The listing builds one solid part. Answer for the finished solid, in the listing's coordinates (mm). Face numbers are marked on the shaded views. A direction names the side the tool comes from. Round coordinates to 2 decimals unless told otherwise and drop trailing zeros. Write each loop counter-clockwise with the first axis right and the second up, starting at its lowest first coordinate (ties: lowest second). Pieces come first, ordered by that corner, then holes.
from build123d import *
from build123d.topology import SkipClean

# Parameters (mm, degrees)
EXTRUDE_1_DEPTH = 4
SKETCH_2_R      = 3
SKETCH_2_R_2    = 1.05
EXTRUDE_2_DEPTH = 3
EXTRUDE_START   = -7
SKETCH_3_R      = 2
EXTRUDE_3_DEPTH = 7


with BuildPart() as part:
    # Эскиз1 → Бобышка-Вытянуть1 (new body)
    with BuildSketch(Plane.XY):
        with BuildLine():
            Line((14.386891947, -11.67121845), (-1.44161316, -9.187586816))
            ThreePointArc((-1.44161316, -9.187586816), (-8.668259234, 3.369166345), (5.141479906, 7.74952801))
            Line((5.141479906, 7.74952801), (18.492476869, -1.108286623))
            ThreePointArc((18.492476869, -1.108286623), (20.691973654, -8.042526113), (14.386891947, -11.67121845))
        make_face()
        with BuildLine():
            Line((3.482938001, 5.249680265), (16.833934964, -3.608134368))
            ThreePointArc((16.833934964, -3.608134368), (17.895760998, -6.95569826), (14.85192845, -8.707480768))
            Line((14.85192845, -8.707480768), (-0.976576656, -6.223849133))
            ThreePointArc((-0.976576656, -6.223849133), (-5.872046578, 2.282338492), (3.482938001, 5.249680265))
        make_face(mode=Mode.SUBTRACT)
    extrude(amount=EXTRUDE_1_DEPTH)

    # Эскиз2 → Бобышка-Вытянуть2 (add)
    with SkipClean():  # the faces are left unmerged after this step: merging them gives an invalid solid
        with BuildSketch(Plane.XY.offset(4)):
            with BuildLine():
                Line((-1.44161316, -9.187586816), (14.386891947, -11.67121845))
                ThreePointArc((14.386891947, -11.67121845), (20.691973654, -8.042526113), (18.492476869, -1.108286623))
                Line((18.492476869, -1.108286623), (5.141479906, 7.74952801))
                ThreePointArc((5.141479906, 7.74952801), (-8.668259234, 3.369166345), (-1.44161316, -9.187586816))
            make_face()
            Circle(SKETCH_2_R, mode=Mode.SUBTRACT)
            with Locations((6.897324552, -2.680842038)):
                Circle(SKETCH_2_R_2, mode=Mode.SUBTRACT)
            with Locations((9.693537208, -3.767669891)):
                Circle(SKETCH_2_R_2, mode=Mode.SUBTRACT)
            with Locations((12.489749864, -4.854497744)):
                Circle(SKETCH_2_R_2, mode=Mode.SUBTRACT)
            with Locations((15.28596252, -5.941325597)):
                Circle(SKETCH_2_R_2, mode=Mode.SUBTRACT)
        extrude(amount=EXTRUDE_2_DEPTH)

    # Эскиз3 → Бобышка-Вытянуть3 (add)
    with SkipClean():  # the faces are left unmerged after this step: merging them gives an invalid solid
        with BuildSketch(Plane.XY.offset(7).offset(EXTRUDE_START)):
            with BuildLine():
                Line((18.492476869, -1.108286623), (24.987431668, -4.371825212))
                ThreePointArc((24.987431668, -4.371825212), (27.402884029, -10.650912961), (21.380978505, -13.650580764))
                Line((21.380978505, -13.650580764), (14.386891947, -11.67121845))
                ThreePointArc((14.386891947, -11.67121845), (20.691973654, -8.042526113), (18.492476869, -1.108286623))
            make_face()
            with Locations((22.742529602, -8.839533206)):
                Circle(SKETCH_3_R, mode=Mode.SUBTRACT)
        extrude(amount=EXTRUDE_3_DEPTH)


solid = part.part
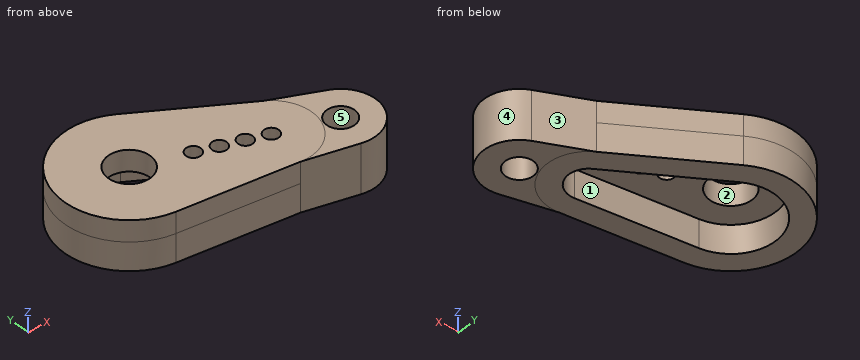
1. Section C-C on z = 2.25 is taken. Determine the outline of the cut face in (x, y).
Geometry says:
outline: (-1.44, -9.19) - (14.39, -11.67) - (21.38, -13.65) arc R5 ccw to (24.99, -4.37) - (18.49, -1.11) - (5.14, 7.75) arc R9.3 ccw (long way) to start; hole (-0.98, -6.22) - (14.85, -8.71) arc R2.8 ccw to (16.83, -3.61) - (3.48, 5.25) arc R6.3 ccw (long way) to start; hole circle Ø4 at (22.74, -8.84)
2. A tool of negligible diameter and unlimited length cuts with its end or side. For the marked faces 1 and 2, from which of +Z, -Z, +X, -X, +Y, -Y can it reach the whole face along a straight path? Write none if from no direction.
Geometry says:
face 1: -Z
face 2: +Z, -Z
3. Section B-B on y = -8 is taken. Determine the outline of the cut face in (x, z).
Geometry says:
outline: (-4.74, 0) - (10.34, 0) - (10.34, 4) - (17.18, 4) - (17.18, 0) - (20.93, 0) - (20.93, 7) - (-4.74, 7) - close; (24.56, 0) - (27.67, 0) - (27.67, 7) - (24.56, 7) - close
4. Given pin 1 (2.5 mm diameter, centred on x = 12.49, y = -4.85, fed in from -Z); pin 2 (1.7 mm diameter, centred on x = 9.69, y = -3.77, fed in from -Z); pin 3 (1.5 mm diameter, centred on x = 13, z = 2, fed in from +Y); pin 4 (1 mm diameter, centred on x = 11, z = 5.5, fed in from -Y), each flat-ended and moving along its own axis, determine where each tip first touches the part or whether it passes through.
Geometry says:
pin 1: stops at z = 4
pin 2: passes through
pin 3: stops at y = 3.03
pin 4: stops at y = -11.22
5. Straight lines are drawn through the part: line 1 along X through (y, z) = (-4.75, 1.25); line 2 along X through (y, z) = (-5.5, 2); line 3 along Z through (x, y) = (7.5, -5.75). For each, find the intervals that lie inside material, in ascending order.
Geometry says:
line 1: x = -8 to -4.14, 17.82 to 25.62
line 2: x = -7.5 to -3.07, 18.05 to 26.46
line 3: z = 4 to 7
6. Section A-A on x = 0 is taken. Determine the outline of the cut face in (y, z), plus the area to 3 significant figures.
Geometry says:
outline: (-9.41, 0) - (-6.38, 0) - (-6.38, 4) - (-3, 4) - (-3, 7) - (-9.41, 7) - close; (3, 4) - (6.3, 4) - (6.3, 0) - (9.3, 0) - (9.3, 7) - (3, 7) - close
area: 62.3 mm2
7. Section D-D on x = 19 is taken. Determine the outline of the cut face in (y, z).
Geometry says:
outline: (-12.98, 0) - (-1.36, 0) - (-1.36, 7) - (-12.98, 7) - close
8. For a pull along Y with two mould halves and no side action, classify the marked faces 3, 4 and 5 as released by +Y, released by -Y, zero draft, split by the parting line, or undercut.
Geometry says:
face 3: released by +Y
face 4: split by the parting line
face 5: undercut
